Read the model definition and answer for the solid it produces. Units are mm, in the model's axes. Round coordinates to 2 decimals unless told otherwise and drop trailing zeros. Loops run counter-clockwise (first coordinate to the right, second up) from the corner with the lowest first, then second, coordinate; pieces in that order, holes last. Notation, with made-up numbers: M -3,59.5 L 1,59.5 A27 ccw 1,89.5 Z; hole C 64,10 d2. An arc over 180 degrees is marked long. Answer as CSV lines item,"result".
Autodesk Inventor part; units mm, degrees
ref_plane "Start Plane" through (0, 0, 0) normal (0, 0, 1) x (1, 0, 0)
ref_plane "End Plane" through (0, 0, 1740) normal (0, 0, 1) x (1, 0, 0)
ref_plane "Work Plane4" through (0, 40, 0) normal (0, -0.7071, -0.7071) x (1, 0, 0)
ref_plane "Start Plane" through (0, 0, 0) normal (0, 0, 1) x (1, 0, 0)
ref_plane "End Plane" through (0, 0, 1740) normal (0, 0, 1) x (1, 0, 0)
sketch "Sketch" plane through (0, 0, 0) normal (0, 0, 1) x (1, 0, 0)
  line L0 (-20, -34) -> (-20, 34)
  line L1 (-14, 40) -> (14, 40)
  line L2 (20, 34) -> (20, -34)
  line L3 (14, -40) -> (-14, -40)
  arc A0 (-20, -34) -> (-14, -40) centre (-14, -34) ccw
  arc A1 (20, 34) -> (14, 40) centre (14, 34) ccw
  arc A2 (-14, 40) -> (-20, 34) centre (-14, 34) ccw
  arc A3 (14, -40) -> (20, -34) centre (14, -34) ccw
  arc A4 (-14, 37) -> (-17, 34) centre (-14, 34) ccw
  line L4 (-14, 37) -> (14, 37)
  arc A5 (17, 34) -> (14, 37) centre (14, 34) ccw
  line L5 (17, 34) -> (17, -34)
  arc A6 (14, -37) -> (17, -34) centre (14, -34) ccw
  line L6 (14, -37) -> (-14, -37)
  arc A7 (-17, -34) -> (-14, -37) centre (-14, -34) ccw
  line L7 (-17, -34) -> (-17, 34)
  line L8 (0, 57.7397) -> (0, -57.7397) construction
  line L9 (-29.7397, 0) -> (29.7397, 0) construction
  dimension "d7" = 6
  dimension "d9" = 40
  dimension "d11" = 80
  dimension "d12" = 3
  dimension "d15" = 20
  dimension "d16" = 40
extrude "Body" add sketch "Sketch" along normal up to surface (1740 mm away) from surface at 0
sketch "Sketch3" plane through (0, 0, 0) normal (0, 0, 1) x (1, 0, 0)
  line L0 (0, 0) -> (10, 0)
ref_plane "Work Plane3" through (0, 0, 0) normal (0, -1, 0) x (1, 0, 0)
ref_plane "Work Plane4" through (0, 40, 0) normal (0, -0.7071, -0.7071) x (1, 0, 0)
split "Split1" plane through (0, 40, 0) removes the side toward (0, -0.7071, -0.7071)
ref_plane "Work Plane5" through (0, 40, 1740) normal (0, -0.7071, 0.7071) x (1, 0, 0)
split "Split2" plane through (0, 40, 1740) removes the side toward (0, -0.7071, 0.7071)
sketch "Sketch4" plane through (0, 0, 0) normal (0, -1, 0) x (1, 0, 0)
  line L0 (-2, 0) -> (12, 0)
  line L1 (-2, 1740) -> (12, 1740)
  dimension "d18" = 1740
equation "\"d7\" = G_IR"
equation "\"d9\" = G_W"
equation "\"d11\" = G_H"
equation "\"d12\" = G_T"
equation "\"d15\" = 0.5 * d9"
equation "\"d16\" = 0.5 * d11"
equation "\"d3\" = G_L"
equation "\"G_W\" = 40"
equation "\"G_H\" = 80"
equation "\"G_T\" = 3"
equation "\"G_IR\" = 6"
equation "\"G_L\" = d18"
equation "\"G_OFFSET_START\" = 0"
equation "\"G_OFFSET_END\" = 0"
properties part number "ISO 10799-2 - 80x40x3 - 1740" material "Stainless Steel"
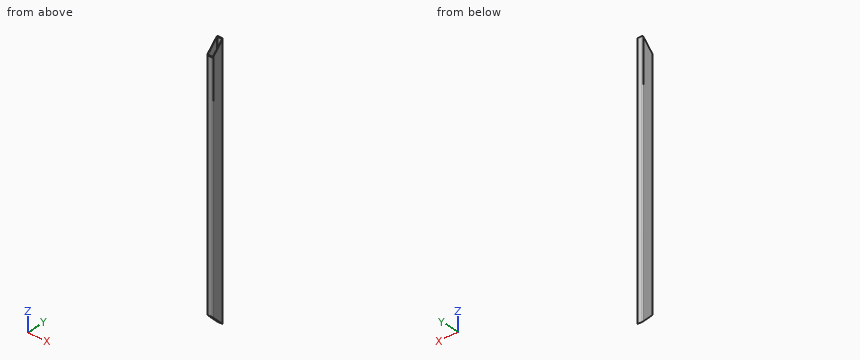
1) Find section A-A, the plane y = -17. Give the vertices of the cut face in (x, z).
Evaluation:
outline,"M -20,57 L -17,57 L -17,1683 L -20,1683 Z; M 17,57 L 20,57 L 20,1683 L 17,1683 Z"
2) Straight lines are drawn through the part: line 1 (Y direction, x = 10, z = 143); line 2 (X direction, y = 33.5, z = 734.5); line 3 (Y direction, x = 15, z = 421). For each, find the intervals that lie inside material, in ascending order.
Evaluation:
line 1,"y = -40 to -37, 37 to 40"
line 2,"x = -20 to -17, 17 to 20"
line 3,"y = -39.92 to -36.83, 36.83 to 39.92"
3) Find section C-C, the plane z = 226. Give the vertices of the cut face in (x, y), then the cut area to 3 significant figures.
Evaluation:
outline,"M -20,-34 A6 ccw -14,-40 L 14,-40 A6 ccw 20,-34 L 20,34 A6 ccw 14,40 L -14,40 A6 ccw -20,34 Z; hole M -17,-34 A3 ccw -14,-37 L 14,-37 A3 ccw 17,-34 L 17,34 A3 ccw 14,37 L -14,37 A3 ccw -17,34 Z"
area,"661 mm^2"
4) Each of these flat-tipped pins is pushed along its axis until it touches: P1, Ø6, axis at x = 15.5, y = 21, coming from the -Z side; P2, Ø1.5, axis at x = 16, z = 1082.5, coming from the +Y side. Where does it stop, or does it pass through?
Evaluation:
P1,"stops at z = 16.4"
P2,"stops at y = 39.87"
5) Find section B-B, the plane x = 1.5. Give the vertices of the cut face in (y, z).
Evaluation:
outline,"M -40,80 L -37,77 L -37,1663 L -40,1660 Z; M 37,3 L 40,0 L 40,1740 L 37,1737 Z"
